Part print with two shaded views. Sizes in mm from the minimum x, y, z corner. A direction names the side the tool comes from. Coordinates: 2 decimals unless noted, no trailing zeros. Loops run counter-clockwise (first coordinate to the right, second up) from the corner with the lowest first, then second, coordinate; pieces in that order, holes last.
Item 1: Cut at B-B (z = 6). List the corners of the cut face in (x, y).
Item 2: Drill centre lines: line 1 along X through (y, z) = (17.6, 6); line 2 along Z through (x, y) = (14, 17.05); line 3 along X through (y, z) = (14, 3.75). Where is each one in solid material? Low to high.
Item 3: Flat gauge pins, fed straight in: pin 1 (0.7 mm diameter, centred on y = 0.5, z = 4, fed in from -X); pin 2 (1.6 mm diameter, centred on y = 1, z = 4.5, fed in from +X). Where does each tip first touch, or does it go through?
Item 4: Cut at A-A (x = 14). List the corners of the cut face in (y, z).
Item 5: 3-axis set-ups, long thin cutter, end or side, ignore diameter. For the marked faces 1 and 2: which of +Z, -Z, +X, -X, +Y, -Y reach the whole face in a straight line?
Item 6: Cut at C-C (y = 7). List the corners of the cut face in (x, z) (1 decimal), and give its area (3 significant figures).
Item 7: Mould opens along Y. For the marked faces 3, 4 and 5 say: released by +Y, released by -Y, zero draft, split by the parting line, or undercut.
Item 8: Cut at D-D (z = 11.25). List the corners of the cut face in (x, y).
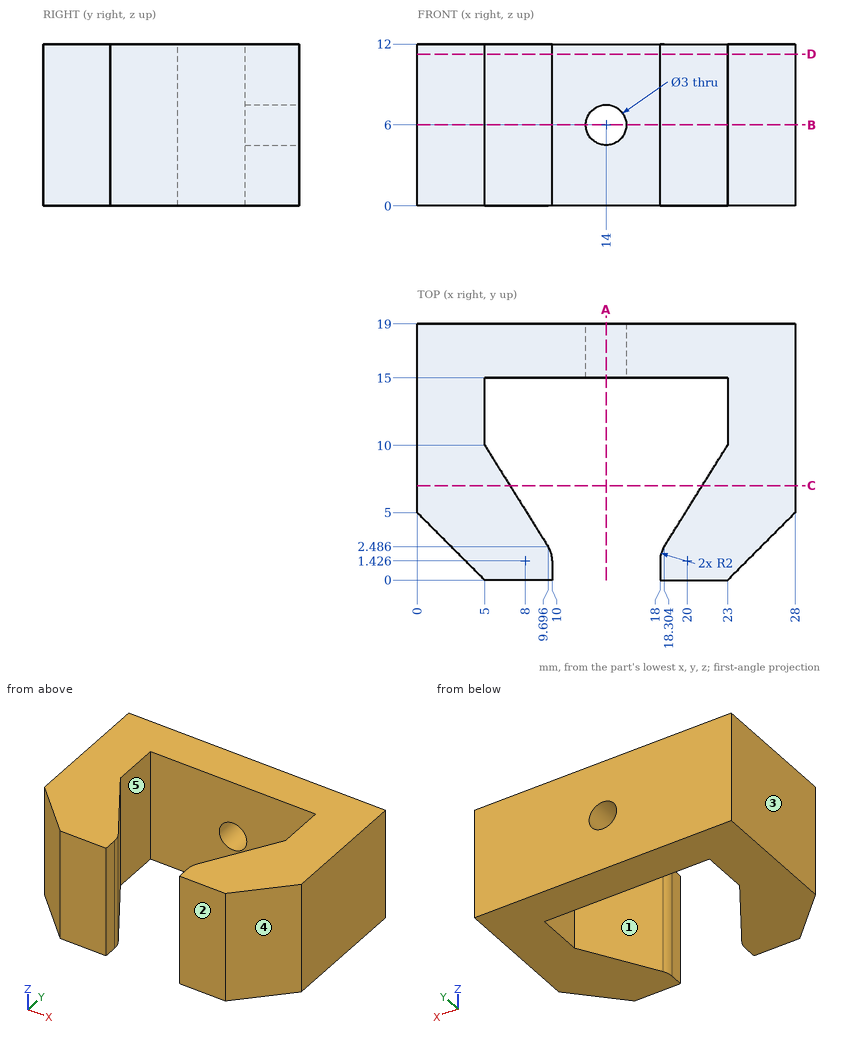
Filled sheet:
1. outline: (0, 5) - (5, 0) - (10, 0) - (10, 1.43) arc R2 ccw to (9.7, 2.49) - (5, 10) - (5, 15) - (12.5, 15) - (12.5, 19) - (0, 19) - close; (15.5, 15) - (23, 15) - (23, 10) - (18.3, 2.49) arc R2 ccw to (18, 1.43) - (18, 0) - (23, 0) - (28, 5) - (28, 19) - (15.5, 19) - close
2. line 1: x = 0 to 12.5, 15.5 to 28
2. line 2: z = 0 to 4.5, 7.5 to 12
2. line 3: x = 0 to 5, 23 to 28
3. pin 1: stops at x = 4.15
3. pin 2: stops at x = 24.8
4. outline: (15, 0) - (19, 0) - (19, 4.5) - (15, 4.5) - close; (15, 7.5) - (19, 7.5) - (19, 12) - (15, 12) - close
5. face 1: +Z, -Z
5. face 2: +Z, -Z, +X, -X, -Y
6. outline: (0, 0) - (6.9, 0) - (6.9, 12) - (0, 12) - close; (21.1, 0) - (28, 0) - (28, 12) - (21.1, 12) - close
6. area: 165 mm2
7. face 3: zero draft
7. face 4: released by -Y
7. face 5: undercut
8. outline: (0, 5) - (5, 0) - (10, 0) - (10, 1.43) arc R2 ccw to (9.7, 2.49) - (5, 10) - (5, 15) - (23, 15) - (23, 10) - (18.3, 2.49) arc R2 ccw to (18, 1.43) - (18, 0) - (23, 0) - (28, 5) - (28, 19) - (0, 19) - close
